Model file for the job. Use its own axes, mm. Face numbers are marked on the shaded views. A direction names the side the tool comes from. Round coordinates to 2 decimals unless told otherwise and drop trailing zeros. Loops run counter-clockwise (first coordinate to the right, second up) from the corner with the lowest first, then second, coordinate; pieces in that order, holes last. Notation, with made-up numbers: M -4,49.25 L 26,49.25 A22 cw 26,74.25 Z; hole C 60.5,-29 d11. An arc over 180 degrees is marked long. Use a Markdown table: item, result. Add a question column.
Q1. Tool access for the marked faces 1, 2, 3 and 4: list every direction of +Z, -Z, +X, -X, +Y, -Y with a clear straight run to the whole face (end or side of a thin tool).
Q2. Probe line 1 (X direction, y = 1.75, z = -3); line 2 (X direction, y = 8.75, z = -9); line 3 (X direction, y = 2.75, z = -18). List the from-to ranges inside material, lowest first. Write a range as from..to.
Q3. Cut at A-A (z = -3). Give the cut face in (x, y), plus the area to 3 significant figures.
Q4. Mould opens along X. For the marked faces 5, 6, 7 and 8 say: +X half, -X half, draft (parallel to the pull), parting line (faces both ways), or undercut.
Q5. Cut at C-C (z = -21.5). Give the cut face in (x, y), plus the area to 3 significant figures.
Q6. Cut at D-D (x = 37). Give the cut face in (y, z), plus the area to 4 significant figures.
Q7. Pin check, flat tips, straight feed: pin 1 (4 mm diameter, centred on y = 5.5, z = 1, fed in from +X); pin 2 (2 mm diameter, centred on x = 26.5, z = -2.5, fed in from -Y); pin 3 (3.5 mm diameter, centred on x = 7.5, y = 4.5, fed in from +Z); pin 4 (5 mm diameter, centred on x = 14, z = -13.5, fed in from +Y). Stop position of each tip, or through.
Q8. Cut at B-B (x = 22). Give the cut face in (y, z).
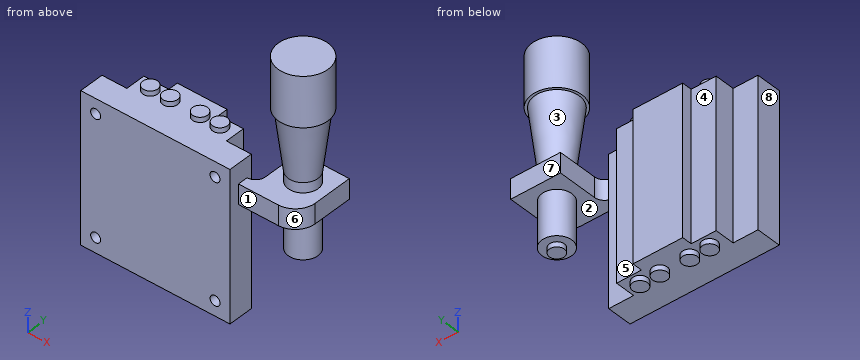
from build123d import *

# Parameters (mm, degrees)
SKETCH_2_W          = 30
SKETCH_2_H          = 30
EXTRUDE_1_DEPTH     = 5
SKETCH_3_R          = 1
CUT_EXTRUDE_1_DEPTH = 3
EXTRUDE_2_DEPTH     = 30
SKETCH_6_W          = 15
SKETCH_6_H          = 2
EXTRUDE_3_DEPTH     = 8
SKETCH_7_W          = 10
SKETCH_7_H          = 4
EXTRUDE_4_DEPTH     = 10
SKETCH_10_W         = 8
SKETCH_10_H         = 2
CUT_EXTRUDE_2_DEPTH = 7
SKETCH_11_W         = 8
SKETCH_11_H         = 2
CUT_EXTRUDE_3_DEPTH = 4
SKETCH_12_W         = 4
SKETCH_12_H         = 2
EXTRUDE_5_DEPTH     = 4
FILLET_1_R          = 4
FILLET_2_R          = 2
SKETCH_13_R         = 1.5
EXTRUDE_6_DEPTH     = 1
EXTRUDE_START       = 1
SKETCH_14_R         = 1.5
EXTRUDE_7_DEPTH     = 1


with BuildPart() as part:
    # Эскиз2 → Бобышка-Вытянуть1 (new body)
    with BuildSketch(Plane(origin=(0, 0, 0), x_dir=(1, 0, 0), z_dir=(0, 1, 0))):
        with Locations((15, 15)):
            Rectangle(SKETCH_2_W, SKETCH_2_H)
    extrude(amount=EXTRUDE_1_DEPTH)

    # Эскиз3 → Вырез-Вытянуть1 (cut)
    with BuildSketch(Plane.XZ):
        with Locations(Location((27, -3, 0), (0, 0, 270))):
            Circle(SKETCH_3_R)
        with Locations(Location((27, -27, 0), (0, 0, 270))):
            Circle(SKETCH_3_R)
        with Locations(Location((3, -27, 0), (0, 0, 270))):
            Circle(SKETCH_3_R)
        with Locations(Location((3, -3, 0), (0, 0, 270))):
            Circle(SKETCH_3_R)
    extrude(amount=-CUT_EXTRUDE_1_DEPTH, mode=Mode.SUBTRACT)

    # Эскиз5 → Бобышка-Вытянуть2 (add)
    with BuildSketch(Plane.XY):
        Polygon((10, 9), (5, 9), (5, 5), (25, 5), (25, 9), (20, 9), (20, 11), (10, 11), align=None)
    extrude(amount=-EXTRUDE_2_DEPTH)

    # Эскиз6 → Бобышка-Вытянуть3 (add)
    with BuildSketch(Plane(origin=(30, 0, 0), x_dir=(0, 0, -1), z_dir=(1, 0, 0))):
        with Locations((7.5, 3)):
            Rectangle(SKETCH_6_W, SKETCH_6_H)
    extrude(amount=EXTRUDE_3_DEPTH)

    # Эскиз7 → Бобышка-Вытянуть4 (add)
    with BuildSketch(Plane(origin=(0, 4, 0), x_dir=(1, 0, 0), z_dir=(0, 1, 0))):
        with Locations((37, 6)):
            Rectangle(SKETCH_7_W, SKETCH_7_H)
    extrude(amount=EXTRUDE_4_DEPTH)

    # Эскиз9 → Повернуть1 (revolve)
    with BuildSketch(Plane.ZY.offset(-37), mode=Mode.PRIVATE) as revolve_1_sk:
        Polygon((20.2, 9), (20.2, 14), (10.2, 14), (10.2, 13.5), (-2, 12), (-17, 12), (-17, 10.5), (-18, 10.5), (-18, 9), align=None)
    revolve(revolve_1_sk.sketch.rotate(Axis((37, 9, -4), (0, 0, 1)), 90), axis=Axis((37, 9, -4), (0, 0, 1)))

    # Эскиз10 → Вырез-Вытянуть2 (cut)
    with BuildSketch(Plane(origin=(0, 0, -15), x_dir=(-1, 0, 0), z_dir=(0, 0, -1))):
        with Locations((-34, 3)):
            Rectangle(SKETCH_10_W, SKETCH_10_H)
    extrude(amount=-CUT_EXTRUDE_2_DEPTH, mode=Mode.SUBTRACT)

    # Эскиз11 → Вырез-Вытянуть3 (cut)
    with BuildSketch(Plane.XY):
        with Locations((34, 3)):
            Rectangle(SKETCH_11_W, SKETCH_11_H)
    extrude(amount=-CUT_EXTRUDE_3_DEPTH, mode=Mode.SUBTRACT)

    # Эскиз12 → Бобышка-Вытянуть5 (add)
    with BuildSketch(Plane(origin=(38, 0, 0), x_dir=(0, 0, -1), z_dir=(1, 0, 0))):
        with Locations((6, 3)):
            Rectangle(SKETCH_12_W, SKETCH_12_H)
    extrude(amount=EXTRUDE_5_DEPTH)

    # Скругление1
    fillet_1_edges = [part.edges().sort_by_distance(p)[0] for p in [
        (42, 2, -6),
    ]]
    fillet(fillet_1_edges, radius=FILLET_1_R)

    # Скругление2
    fillet_2_edges = [part.edges().sort_by_distance(p)[0] for p in [
        (32, 4, -6),
    ]]
    fillet(fillet_2_edges, radius=FILLET_2_R - 0.0001)  # a hair under: the kernel refuses the full size

    # Эскиз13 → Бобышка-Вытянуть6 (add)
    with BuildSketch(Plane.XY):
        with Locations(Location((8, 7, 0), (0, 0, 180))):
            Circle(SKETCH_13_R)
        with Locations(Location((12, 7, 0), (0, 0, 180))):
            Circle(SKETCH_13_R)
        with Locations(Location((22, 7, 0), (0, 0, 180))):
            Circle(SKETCH_13_R)
        with Locations(Location((18, 7, 0), (0, 0, 180))):
            Circle(SKETCH_13_R)
    extrude(amount=EXTRUDE_6_DEPTH)

    # Эскиз14 → Бобышка-Вытянуть7 (add)
    with BuildSketch(Plane(origin=(0, 0, -30), x_dir=(-1, 0, 0), z_dir=(0, 0, -1)).offset(EXTRUDE_START)):
        with Locations((-8, 7)):
            Circle(SKETCH_14_R)
        with Locations((-12, 7)):
            Circle(SKETCH_14_R)
        with Locations((-18, 7)):
            Circle(SKETCH_14_R)
        with Locations((-22, 7)):
            Circle(SKETCH_14_R)
    extrude(amount=-EXTRUDE_7_DEPTH)


solid = part.part
Checked values:
| question | item | result |
|---|---|---|
| 1 | face 1 | +Z, -Z, +X, -Y |
| 1 | face 2 | -Z |
| 1 | face 3 | none |
| 1 | face 4 | +Z, -Z, -X, +Y |
| 2 | line 1 | x = 0..2, 4..26, 28..30 |
| 2 | line 2 | x = 5..25, 34.01..39.99 |
| 2 | line 3 | x = 0..30 |
| 3 | outline | M 0,0 L 2,0 L 2,3 L 4,3 L 4,0 L 26,0 L 26,3 L 28,3 L 28,0 L 30,0 L 30,5 L 25,5 L 25,9 L 20,9 L 20,11 L 10,11 L 10,9 L 5,9 L 5,5 L 0,5 Z; C 37,9 d6 |
| 3 | area | 266 mm^2 |
| 4 | face 5 | undercut |
| 4 | face 6 | +X half |
| 4 | face 7 | draft |
| 4 | face 8 | -X half |
| 5 | outline | M 0,0 L 30,0 L 30,5 L 25,5 L 25,9 L 20,9 L 20,11 L 10,11 L 10,9 L 5,9 L 5,5 L 0,5 Z |
| 5 | area | 250 mm^2 |
| 6 | outline | M 2,-8 L 6,-8 L 6,-17 L 7.5,-17 L 7.5,-18 L 10.5,-18 L 10.5,-17 L 12,-17 L 12,-8 L 14,-8 L 14,-4 L 12,-4 L 12,-2 L 13.5,10.2 L 14,10.2 L 14,20.2 L 4,20.2 L 4,10.2 L 4.5,10.2 L 6,-2 L 6,-4 L 2,-4 Z |
| 6 | area | 308.5 mm^2 |
| 7 | pin 1 | stops at x = 40.05 |
| 7 | pin 2 | stops at y = 0 |
| 7 | pin 3 | stops at z = 1 |
| 7 | pin 4 | stops at y = 11 |
| 8 | outline | M 0,-30 L 5.5,-30 L 5.5,-31 L 8.5,-31 L 8.5,-30 L 9,-30 L 9,0 L 8.5,0 L 8.5,1 L 5.5,1 L 5.5,0 L 0,0 Z |
